from build123d import *

# Parameters (mm, degrees)
PAD_DEPTH    = 3
SKETCH001_R  = 1.5
PAD001_DEPTH = 6


with BuildPart() as part:
    # Sketch → Pad (new body)
    with BuildSketch(Plane.XY):
        Polygon((-6.25, 33), (-6.25, -33), (17.25, -33), (17.25, -11.5), (6.25, -11.5), (6.25, 33), (4, 33), (4, 43), (-4, 43), (-4, 33), align=None)
    extrude(amount=PAD_DEPTH)

    # Sketch001 → Pad001 (join, symmetric)
    with BuildSketch(Plane.YZ):
        with Locations((40, 1.5)):
            Circle(SKETCH001_R)
    extrude(amount=PAD001_DEPTH, both=True)


solid = part.part
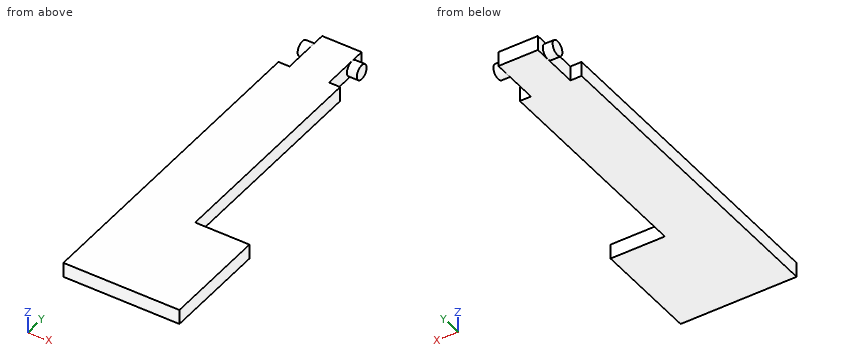
The listing builds one solid part. Answer for the finished solid, in the listing's coordinates (mm). Round coordinates to 2 decimals unless told otherwise and drop trailing zeros. Order: outer loops, then holes, each group sorted by start corner. A loop starts at its lowest first (then second) coordinate and runs counter-clockwise, first axis right, second up. Notation, with made-up numbers: (85.5, -2.75) -> (103.5, -2.75) arc R21 cw to (103.5, 21.25) -> close; hole circle Ø2 at (-38.75, 32). An arc over 180 degrees is marked (long way). Write each question's results on one line, items separated by ' | '. Start each with the question number.
Q1. Find section B-B (y = 10). Determine the outline of the cut face in (x, z).
Q2. Find section C-C (x = 10.5). Determine the outline of the cut face in (y, z).
Q3. Straight lines are drawn through the part: probe 1 along X at (y, z) = (19, 0.85); probe 2 along Y at (x, z) = (10.5, 2.2); probe 3 along X at (y, z) = (39, 0.55). For each, find the intervals that lie inside material, in ascending order. Write a range as from..to.
Q4. Each of these flat-tipped pins is pushed along its axis until it touches: pin 1 (1.5 mm diameter, centred on y = 40, z = 2, fed in from +X); pin 2 (1.5 mm diameter, centred on y = 41, z = 1.5, fed in from -X); pin 3 (1.1 mm diameter, centred on x = 5, z = 1, fed in from +Y). Where does it stop, or does it pass through?
Q5. Find section A-A (z = 1.5). Determine the outline of the cut face in (x, y), then the cut area to 3 significant figures.
Worked answers:
1) outline: (-6.25, 0) -> (6.25, 0) -> (6.25, 3) -> (-6.25, 3) -> close
2) outline: (-33, 0) -> (-11.5, 0) -> (-11.5, 3) -> (-33, 3) -> close
3) probe 1: x = -6.25..6.25 | probe 2: y = -33..-11.5 | probe 3: x = -6..6
4) pin 1: stops at x = 6 | pin 2: stops at x = -6 | pin 3: stops at y = 41.5
5) outline: (-6.25, -33) -> (17.25, -33) -> (17.25, -11.5) -> (6.25, -11.5) -> (6.25, 33) -> (4, 33) -> (4, 38.5) -> (6, 38.5) -> (6, 41.5) -> (4, 41.5) -> (4, 43) -> (-4, 43) -> (-4, 41.5) -> (-6, 41.5) -> (-6, 38.5) -> (-4, 38.5) -> (-4, 33) -> (-6.25, 33) -> close | area: 1,150 mm2
